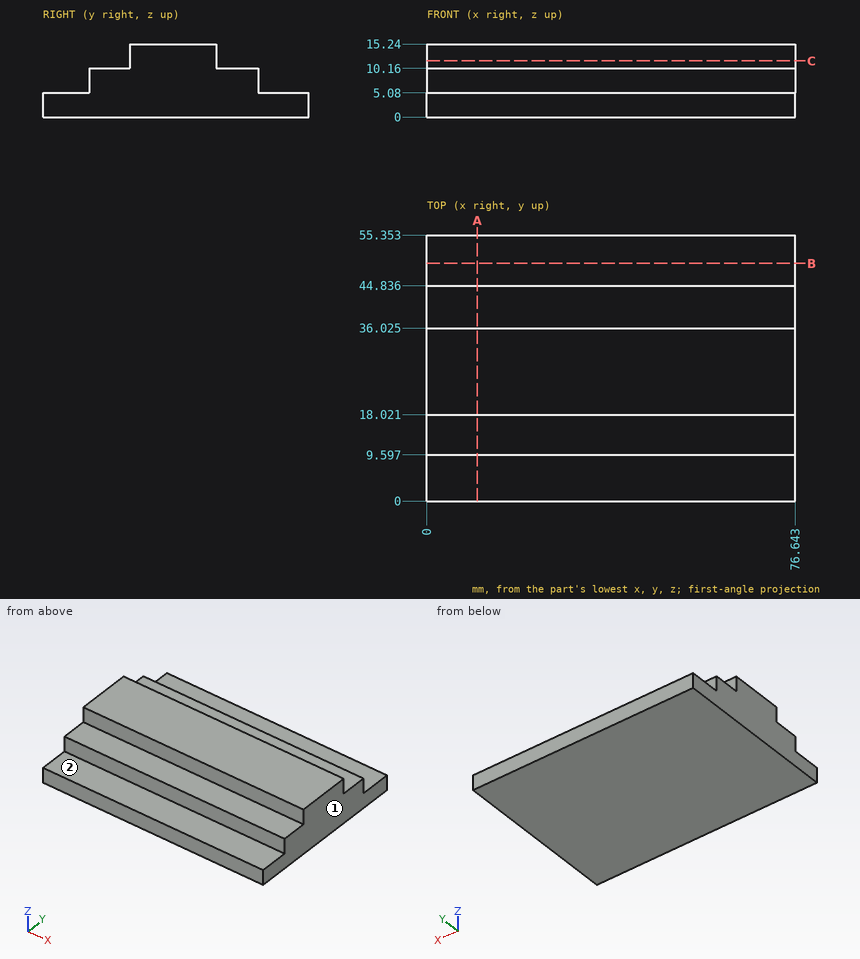
Verification items for this drawing (mm, ordinates from the low corner). A direction names the side the tool comes from. Coordinates: 2 decimals unless noted, no trailing zeros. Loops run counter-clockwise (first coordinate to the right, second up) from the corner with the lowest first, then second, coordinate; pieces in that order, holes last. Notation, with made-up numbers: (-8.5, -29) - (-4.5, -29) arc R15 cw to (-4.5, -18) - close; hole circle Ø4 at (68, 54). An arc over 180 degrees is marked (long way). Answer as a JSON object with one key per item and string values.
(1) Cross-section at C-C, the plane z = 11.75. Record the boundary of the cut face in (x, y) (1 decimal), then the cut area to 3 significant figures.
Response:
{"outline": "(0, 18) - (76.6, 18) - (76.6, 36) - (0, 36) - close", "area": "1,380 mm²"}
(2) Go/stop test with flat-tipped pins: pin 1 Ø1.5 at (x, z) = (30.5, 12.5) entering from +Y (3 decimals); pin 2 Ø5.5 at (x, z) = (39.5, 8) entering from -Y; pin 3 Ø3 at (x, y) = (56.5, 4) entering from +Z. Record where each tip stops, or that it passes through.
Response:
{"pin 1": "stops at y = 36.025", "pin 2": "stops at y = 9.6", "pin 3": "stops at z = 5.08"}
(3) Access from +Z, -Z, +X, -X, +Y, -Y to the whole of each face (thin tool, end or side, straight path). Record for the marked faces 1 and 2.
Response:
{"face 1": "+Z, -Z, +X, +Y, -Y", "face 2": "+Z, +X, -X, -Y"}
(4) Scan lines: line 1 along Z through (x, y) = (4, 50); line 2 along Y through (x, z) = (67, 12) (1 decimal); line 3 along Y through (x, z) = (56, 8). Record each from-to range of solid material in increasing order.
Response:
{"line 1": "z = 0 to 5.08", "line 2": "y = 18 to 36", "line 3": "y = 9.6 to 44.84"}
(5) Cross-section at B-B, the plane y = 49.5. Record the boundary of the cut face in (x, z), then the cut area to 3 significant figures.
Response:
{"outline": "(0, 0) - (76.64, 0) - (76.64, 5.08) - (0, 5.08) - close", "area": "389 mm²"}
(6) Cross-section at A-A, the plane x = 10.5. Record the boundary of the cut face in (y, z) (1 decimal).
Response:
{"outline": "(0, 0) - (55.4, 0) - (55.4, 5.1) - (44.8, 5.1) - (44.8, 10.2) - (36, 10.2) - (36, 15.2) - (18, 15.2) - (18, 10.2) - (9.6, 10.2) - (9.6, 5.1) - (0, 5.1) - close"}
